Source: CAD feature listing. Evaluate the final solid. Frame: model axes, mm. A direction names the side the tool comes from. Give positions to 0.01 mm unless a question says otherwise; leave off trailing zeros. Order: outer loops, then holes, each group sorted by start corner. A loop starts at its lowest first (then second) coordinate and runs counter-clockwise, first axis right, second up. Notation, with made-up numbers: M -36,-33.75 L 0,-33.75 A8 cw 0,-22.75 Z; hole C 35,-18 d4. An arc over 180 degrees is marked long. Answer in a Markdown table with one row per item. Add a question column.
(1) Section query B-B, the plane z = 5. Return loops of the section in (x, y).
(2) Set-up query: faces 4 (the face through (-3, 3, 5)), 5 (the face through (-50, 2, 4)), 6 (the face through (9.647, 1.479, 17.348)), 7 (the face through (-44, 2, 29.5)). Return all of +Z, -Z, +X, -X, +Y, -Y with unobstructed straight access to the full face (end or side cutting, diameter ignored); none if empty.
(3) Section query D-D, the plane z = 22. Return loops of the section in (x, y), plus the area to 3 significant figures.
(4) Pin query (flat end, axial travel): P1, Ø3.5, axis at x = -67.75, z = 18, coming from the +Y side; P2, Ø3.5, axis at x = 9.55, z = 15.1, coming from the +Y side; P3, Ø1.5, axis at y = 1.5, z = 3.5, coming from the +X side; P4, Ø3, axis at y = 3, z = 21, coming from the +X side. Return the tip coordinate at first contact, or that it passes through.
(5) Mould query, pull axis Z, two halves, no side actions, for faces 1 (the face through (-5, 3, 27.5)), 2 (the face through (-5.626, 1.983, 29.528)), 3 (the face through (27, 3, 22)). Classes: pulls with the +Z half, pulls with the -Z half, needs draft (parallel to the pull), parting line crosses it, or undercut.
(6) Section query A-A, the plane x = 28.75. Return loops of the section in (y, z), plus the area to 3 significant figures.
(7) Material intervals for line 1 along X through (y, z) = (1.45, 5); line 2 along X through (y, z) = (2.8, 28.5); line 3 along X through (y, z) = (1.8, 28.5), sorted ascending.
(8) Section query C-C, the plane z = 11.1. Return loops of the section in (x, y).
from build123d import *

# Parameters (mm, degrees)
EXTRUDE_1_DEPTH      = 5
SKETCH_1_20_R        = 1.5
CUT_EXTRUDE_2_DEPTH  = 79.662649968
CUT_EXTRUDE_START    = 5
SKETCH_1_22_R        = 2.25
CUT_EXTRUDE_3_DEPTH  = 2
SKETCH_1_23_R        = 2.6
CUT_EXTRUDE_4_DEPTH  = 2.6
SKETCH_1_24_R        = 1.1
CUT_EXTRUDE_6_DEPTH  = 84.662649968
SKETCH_4_R           = 1.5
CUT_EXTRUDE_7_DEPTH  = 79.662649968
SKETCH_4_3_R         = 2.25
CUT_EXTRUDE_8_DEPTH  = 3
SKETCH_5_W           = 47.701964887
SKETCH_5_H           = 5
EXTRUDE_2_DEPTH      = 2
SKETCH_6_R           = 0.85
CUT_EXTRUDE_9_DEPTH  = 4
SKETCH_1_25_R        = 5
CUT_EXTRUDE_12_DEPTH = 80.434328221
SKETCH_1_26_R        = 3.5
CUT_EXTRUDE_13_DEPTH = 2


with BuildPart() as part:
    # 草图1 → 凸台-拉伸1 (new body)
    with BuildSketch(Plane(origin=(0, 0, 0), x_dir=(1, 0, 0), z_dir=(0, 1, 0))):
        Polygon((-72.75, -7.5), (-72.75, -29.5), (32.75, -29.5), (32.75, -7.5), (0, -7.5), (0, 0), (-50, 0), (-50, -7.5), align=None)
    extrude(amount=EXTRUDE_1_DEPTH)

    # 草图1<20> → 切除-拉伸2 (cut, through all)
    with BuildSketch(Plane(origin=(0, 0, 0), x_dir=(1, 0, 0), z_dir=(0, 1, 0))):
        with Locations(Location((-19.5, -5, 0), (0, 0, 270))):
            Circle(SKETCH_1_20_R)
        with Locations(Location((-5, -5, 0), (0, 0, 270))):
            Circle(SKETCH_1_20_R)
        with Locations(Location((-67.75, -18, 0), (0, 0, 270))):
            Circle(SKETCH_1_20_R)
    extrude(amount=CUT_EXTRUDE_2_DEPTH, mode=Mode.SUBTRACT)

    # 草图1<22> → 切除-拉伸3 (cut)
    with BuildSketch(Plane(origin=(0, 0, 0), x_dir=(1, 0, 0), z_dir=(0, 1, 0)).offset(CUT_EXTRUDE_START)):
        with Locations(Location((-19.5, -5, 0), (0, 0, 270))):
            Circle(SKETCH_1_22_R)
        with Locations(Location((-5, -5, 0), (0, 0, 270))):
            Circle(SKETCH_1_22_R)
        with Locations(Location((-67.75, -18, 0), (0, 0, 270))):
            Circle(SKETCH_1_22_R)
    extrude(amount=-CUT_EXTRUDE_3_DEPTH, mode=Mode.SUBTRACT)

    # 草图1<23> → 切除-拉伸4 (cut)
    with BuildSketch(Plane(origin=(0, 0, 0), x_dir=(1, 0, 0), z_dir=(0, 1, 0)).offset(CUT_EXTRUDE_START)):
        with Locations(Location((25.083939444, -11.1, 0), (0, 0, 270))):
            Circle(SKETCH_1_23_R)
    extrude(amount=-CUT_EXTRUDE_4_DEPTH, mode=Mode.SUBTRACT)

    # 草图1<24> → 切除-拉伸6 (cut, through all)
    with BuildSketch(Plane(origin=(0, 0, 0), x_dir=(1, 0, 0), z_dir=(0, 1, 0)).offset(CUT_EXTRUDE_START)):
        with Locations(Location((28.75, -22, 0), (0, 0, 270))):
            Circle(SKETCH_1_24_R)
        with Locations(Location((25.083939444, -11.1, 0), (0, 0, 270))):
            Circle(SKETCH_1_24_R)
    extrude(amount=-CUT_EXTRUDE_6_DEPTH, mode=Mode.SUBTRACT)

    # 草图4 → 切除-拉伸7 (cut, through all)
    with BuildSketch(Plane.XZ):
        with Locations(Location((9.548035113, 15.1, 0), (0, 0, 270))):
            Circle(SKETCH_4_R)
        with Locations(Location((9.548035113, 26.5, 0), (0, 0, 270))):
            Circle(SKETCH_4_R)
    extrude(amount=-CUT_EXTRUDE_7_DEPTH, mode=Mode.SUBTRACT)

    # 草图4<3> → 切除-拉伸8 (cut)
    with BuildSketch(Plane.XZ):
        with Locations(Location((9.548035113, 15.1, 0), (0, 0, 270))):
            Circle(SKETCH_4_3_R)
        with Locations(Location((9.548035113, 26.5, 0), (0, 0, 270))):
            Circle(SKETCH_4_3_R)
    extrude(amount=-CUT_EXTRUDE_8_DEPTH, mode=Mode.SUBTRACT)

    # 草图5 → 凸台-拉伸2 (add)
    with BuildSketch(Plane.XY.offset(29.5)):
        with Locations((8.899017556, 2.5)):
            Rectangle(SKETCH_5_W, SKETCH_5_H)
    extrude(amount=EXTRUDE_2_DEPTH)

    # 草图6 → 切除-拉伸9 (cut)
    with BuildSketch(Plane.XY.offset(31.5)):
        with Locations((22.75, 2.5)):
            Circle(SKETCH_6_R)
        with Locations((-4.951964887, 2.5)):
            Circle(SKETCH_6_R)
    extrude(amount=-CUT_EXTRUDE_9_DEPTH, mode=Mode.SUBTRACT)

    # 草图1<25> → 切除-拉伸12 (cut, through all)
    with BuildSketch(Plane(origin=(0, 0, 0), x_dir=(1, 0, 0), z_dir=(0, 1, 0))):
        with Locations((35.25, -22)):
            Circle(SKETCH_1_25_R)
    extrude(amount=CUT_EXTRUDE_12_DEPTH, mode=Mode.SUBTRACT)

    # 草图1<26> → 切除-拉伸13 (cut)
    with BuildSketch(Plane(origin=(0, 0, 0), x_dir=(1, 0, 0), z_dir=(0, 1, 0)).offset(CUT_EXTRUDE_START)):
        with Locations((28.75, -22)):
            Circle(SKETCH_1_26_R)
    extrude(amount=-CUT_EXTRUDE_13_DEPTH, mode=Mode.SUBTRACT)


solid = part.part
Values follow:
| question | item | result |
|---|---|---|
| 1 | outline | M -50,0 L -21,0 L -21,3 L -21.75,3 L -21.75,5 L -50,5 Z; M -18,0 L -6.5,0 L -6.5,3 L -7.25,3 L -7.25,5 L -17.25,5 L -17.25,3 L -18,3 Z; M -3.5,0 L 0,0 L 0,5 L -2.75,5 L -2.75,3 L -3.5,3 Z |
| 2 | face 4 | +Y |
| 2 | face 5 | -Z, -X, +Y, -Y |
| 2 | face 6 | -Y |
| 2 | face 7 | +Z, -X, +Y, -Y |
| 3 | outline | M -72.75,0 L 27.65,0 L 27.65,3 L 25.25,3 L 25.25,5 L -72.75,5 Z; M 29.85,0 L 30.25,0 L 30.25,3 L 29.85,3 Z |
| 3 | area | 498 mm² |
| 4 | P1 | stops at y = 3 |
| 4 | P2 | stops at y = 5 |
| 4 | P3 | stops at x = 0 |
| 4 | P4 | stops at x = 30.92 |
| 5 | face 1 | pulls with the +Z half |
| 5 | face 2 | needs draft |
| 5 | face 3 | undercut |
| 6 | outline | M 0,7.5 L 5,7.5 L 5,18.5 L 3,18.5 L 3,20.9 L 0,20.9 Z; M 0,23.1 L 3,23.1 L 3,25.5 L 5,25.5 L 5,31.5 L 0,31.5 Z |
| 6 | area | 99.4 mm² |
| 7 | line 1 | x = -50 to -21, -18 to -6.5, -3.5 to 0 |
| 7 | line 2 | x = -72.75 to -5.75, -4.16 to 8.52, 10.58 to 21.95, 23.55 to 32.75 |
| 7 | line 3 | x = -72.75 to -5.43, -4.47 to 8.52, 10.58 to 22.27, 23.23 to 32.75 |
| 8 | outline | M -72.75,0 L 23.98,0 L 23.98,2.4 L 22.48,2.4 L 22.48,5 L -72.75,5 Z; M 26.18,0 L 32.75,0 L 32.75,5 L 27.68,5 L 27.68,2.4 L 26.18,2.4 Z |
